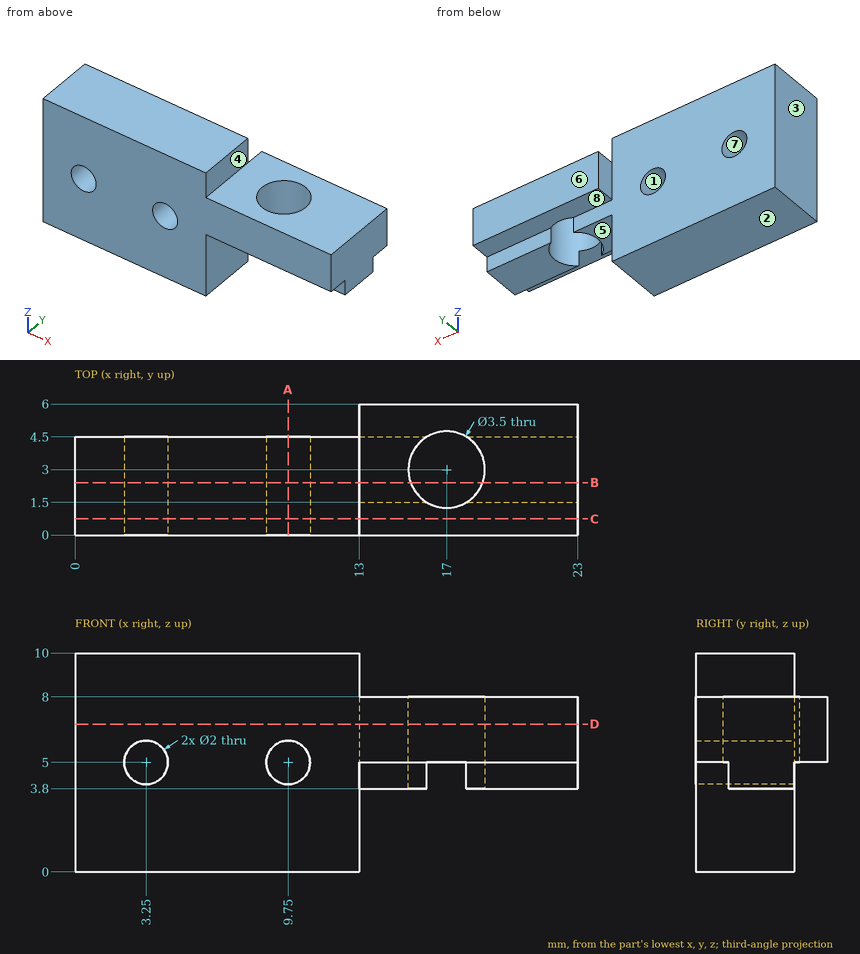
Geometry: see drawing. Coordinates: mm, zero at the bounding-box minimum. A direction names the side the tool comes from. Round coordinates to 2 decimals unless told otherwise and drop trailing zeros. Write each loop counter-clockwise with the first axis right and the second up, starting at its lowest first coordinate (ties: lowest second). Pieces come first, ordered by that corner, then holes.
1) Contact query for flat-ended pins moving along their axis: P1, Ø1.5, axis at x = 15, y = 2.5, coming from the -Z side; P2, Ø1.6, axis at y = 5.5, z = 6.5, coming from the -X side; P3, Ø1.5, axis at x = 9, z = 3.5, coming from the +Y side. Output: stop coordinate, or through.
2) Reachability of the marked faces 4, 5, 6, 7 and 8 from +Z, -Z, +X, -X, +Y, -Y: full face, straight path, thin tool, end or side. Return the list, or none.
3) Cut plane A-A (x = 9.75). Return the cut outline in (y, z).
4) Cut plane B-B (y = 2.4). Return the cut outline in (x, z).
5) Ray query, L1, parallel to X at y = 3.1, z = 5; L2, parallel to Z at x = 9.75, y = 2.15; L3, parallel to X at y = 1.7, z = 5. Return the intervals inside material, ascending.
6) Cut plane D-D (z = 6.75). Return the cut outline in (x, y).
7) Draft query along Z for the marked faces 1, 2 and 3. Return one class per face: pulls with the +Z half, pulls with the -Z half, needs draft (parallel to the pull), parting line crosses it, or undercut.
8) Cut plane C-C (y = 0.75). Return the cut outline in (x, z).
Geometry says:
1. P1: stops at z = 3.8
1. P2: stops at x = 13
1. P3: stops at y = 4.5
2. face 4: +Z, +X, +Y, -Y
2. face 5: -Z, +X, +Y, -Y
2. face 6: +Z, -Z, +X, -X, +Y
2. face 7: +Y, -Y
2. face 8: -Z, +X, -X, +Y
3. outline: (0, 0) - (4.5, 0) - (4.5, 4) - (0, 4) - close; (0, 6) - (4.5, 6) - (4.5, 10) - (0, 10) - close
4. outline: (0, 0) - (13, 0) - (13, 3.8) - (15.36, 3.8) - (15.36, 8) - (13, 8) - (13, 10) - (0, 10) - close; (18.64, 3.8) - (23, 3.8) - (23, 8) - (18.64, 8) - close; hole circle Ø2 at (3.25, 5); hole circle Ø2 at (9.75, 5)
5. L1: x = 0 to 2.25, 4.25 to 8.75, 10.75 to 15.25, 18.75 to 23
5. L2: z = 0 to 4, 6 to 10
5. L3: x = 0 to 2.25, 4.25 to 8.75, 10.75 to 15.83, 18.17 to 23
6. outline: (0, 0) - (23, 0) - (23, 6) - (13, 6) - (13, 4.5) - (0, 4.5) - close; hole circle Ø3.5 at (17, 3)
7. face 1: undercut
7. face 2: pulls with the -Z half
7. face 3: needs draft
8. outline: (0, 0) - (13, 0) - (13, 5) - (23, 5) - (23, 8) - (13, 8) - (13, 10) - (0, 10) - close; hole circle Ø2 at (3.25, 5); hole circle Ø2 at (9.75, 5)
